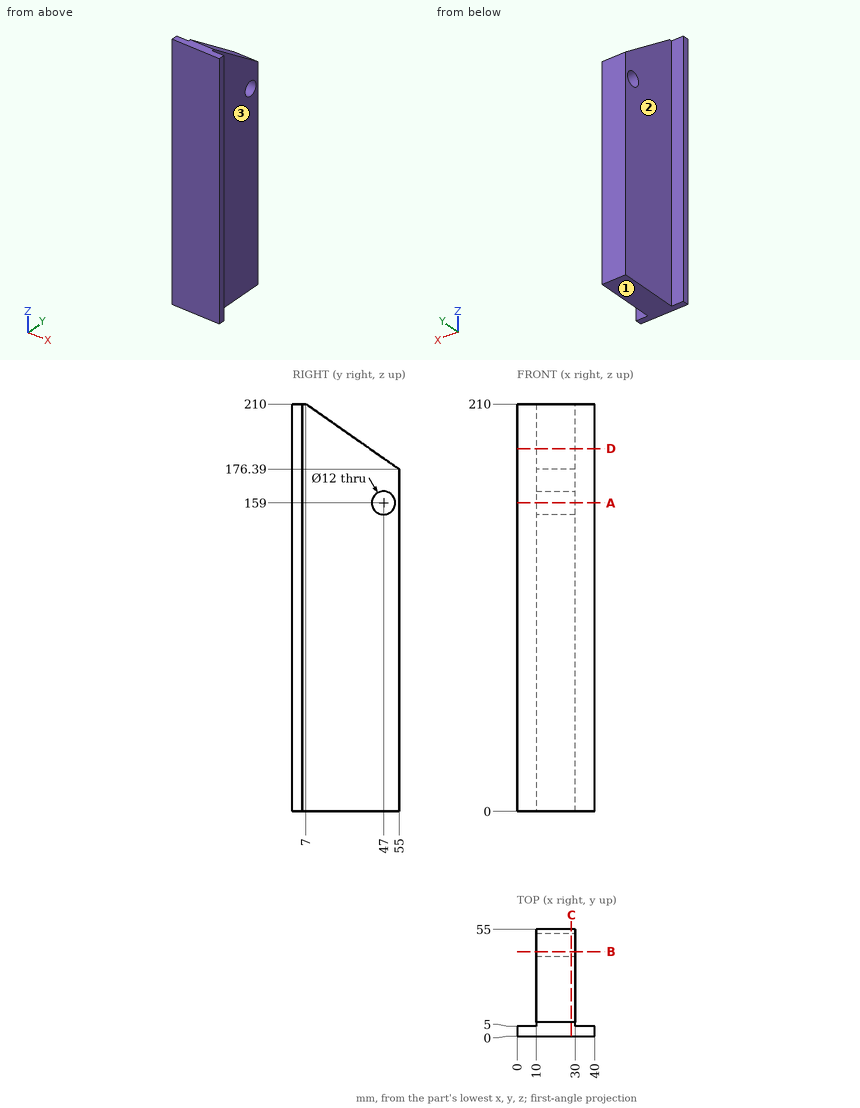
Could you check a few things on this drawing? It's one solid part, dimensions in mm from its lowest x, y, z. A direction names the side the tool comes from. Round coordinates to 2 decimals unless told otherwise and drop trailing zeros. Write each loop counter-clockwise with the first axis right and the second up, starting at its lowest first coordinate (ties: lowest second). Pieces come first, ordered by that corner, then holes. Notation, with made-up numbers: (-20, -31) -> (32, -31) arc R17 cw to (32, -15) -> close; hole circle Ø8 at (52, 50.25). An arc over 180 degrees is marked (long way). One line per item, written item: value.
1) Suppose I cut it at D-D on z = 187. List the corners of the cut face in (x, y) for me.
Filled sheet:
outline: (0, 0) -> (40, 0) -> (40, 5) -> (30, 5) -> (30, 39.85) -> (10, 39.85) -> (10, 5) -> (0, 5) -> close
2) I'm going to push flat-ended pins straight in: pin 1 Ø25 at (y, z) = (25, 150.5) entering from +X; pin 2 Ø8 at (y, z) = (44, 169.5) entering from -X; pin 3 Ø11 at (x, z) = (3.5, 147) entering from +Y. Where does each tip first touch, or does it pass through?
Filled sheet:
pin 1: stops at x = 30
pin 2: stops at x = 10
pin 3: stops at y = 5
3) Suppose I cut it at A-A on z = 159. List the corners of the cut face in (x, y) for me.
Filled sheet:
outline: (0, 0) -> (40, 0) -> (40, 5) -> (30, 5) -> (30, 41) -> (10, 41) -> (10, 5) -> (0, 5) -> close; (10, 53) -> (30, 53) -> (30, 55) -> (10, 55) -> close
4) If I drill on line 1 (Y direction, x = 23.5, z = 159); line 2 (Y direction, x = 32, z = 147); line 3 (X direction, y = 29.5, z = 194), over which ranges is the centre line in solid material (lowest first)? Write a range as [from, to].
Filled sheet:
line 1: y = [0, 41], [53, 55]
line 2: y = [0, 5]
line 3: x = [10, 30]
5) Suppose I cut it at C-C on x = 28. List the corners of the cut face in (y, z) for me, plus the area to 3 significant figures.
Filled sheet:
outline: (0, 0) -> (55, 0) -> (55, 176.39) -> (7, 210) -> (0, 210) -> close; hole circle Ø12 at (47, 159)
area: 10,600 mm2
6) For the marked faces 1, 2 and 3, which set-ups out of +Z, -Z, +X, -X, +Y, -Y let a thin tool reach every point of the face, with its end or its side?
Filled sheet:
face 1: -Z, +X, -X, +Y, -Y
face 2: +Z, -Z, -X, +Y
face 3: +Z, -Z, +X, +Y
7) Suppose I cut it at B-B on y = 43.5. List the corners of the cut face in (x, z) for me, plus the area to 3 significant figures.
Filled sheet:
outline: (10, 0) -> (30, 0) -> (30, 154.13) -> (10, 154.13) -> close; (10, 163.87) -> (30, 163.87) -> (30, 184.44) -> (10, 184.44) -> close
area: 3,490 mm2
